Check sheet for the drawn part. Datum: minimum x, y, z corner. Units: mm. Coordinates: 2 decimals unless noted, no trailing zeros. Order: outer loops, then holes, each group sorted by start corner. A loop starts at its lowest first (then second) coordinate and runs counter-clockwise, first axis right, second up. Notation, with made-up numbers: (-5.75, 84.25) - (36.25, 84.25) arc R20 ccw to (36.25, 116.25) - close; hole circle Ø7 at (-19, 5.5). An arc over 180 degrees is marked (long way). Answer as CSV lines item,"result". Start each with the question number.
1. Go/stop test with a flat-tipped pin: pin 1 (6 mm diameter, centred on x = 177.5, y = 74, fed in from +Z). Record where the tip stops, or that it passes through.
2. Material ranges on L1, parallel to Y at x = 281, z = 3.75; L2, parallel to Z at x = 282, y = 84.5, recorded low to high. Write a range as [from, to].
3. Section check A-A (z = 16.75). Record the cut outline in (x, y).
4. Section check B-B (x = 411.5). Record the cut outline in (y, z).
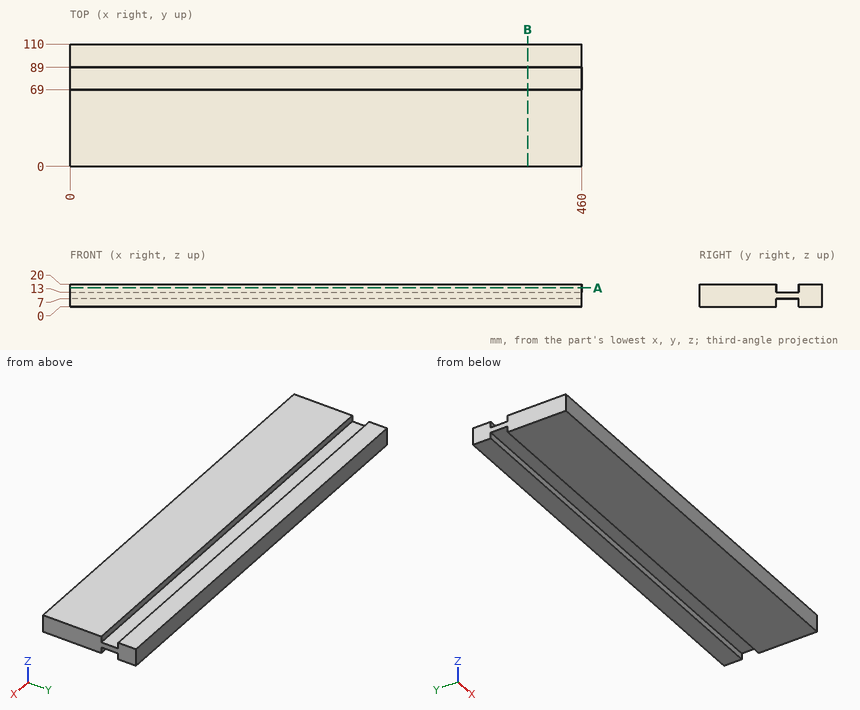
Evaluation:
1,pin 1,"stops at z = 13"
2,L1,"y = [0, 69], [89, 110]"
2,L2,"z = [7, 13]"
3,outline,"(0, 0) - (460, 0) - (460, 69) - (0, 69) - close; (0, 89) - (460, 89) - (460, 110) - (0, 110) - close"
4,outline,"(0, 0) - (69, 0) - (69, 7) - (89, 7) - (89, 0) - (110, 0) - (110, 20) - (89, 20) - (89, 13) - (69, 13) - (69, 20) - (0, 20) - close"
